Here's how the part is built. I have some questions about the finished solid (model axes, mm). Face numbers are marked on the shaded views. Coordinates: 2 decimals unless noted, no trailing zeros. Loops run counter-clockwise (first coordinate to the right, second up) from the corner with the lowest first, then second, coordinate; pieces in that order, holes last.
```python
from build123d import *

# Parameters (mm, degrees)
F1_DEPTH = 19.5
F3_R     = 3
F4_DEPTH = 60.866634
F3_R_2   = 5
F5_DEPTH = 40.43


with BuildPart() as f1:
    # F0 (on Front) → F1 (new body)
    with BuildSketch(Plane.XZ):
        with BuildLine():
            Line((-53.260562, 35.884366), (-67.116969, 27.884366))
            ThreePointArc((-67.116969, 27.884366), (0, -10.865634), (67.116969, 27.884366))
            Line((67.116969, 27.884366), (53.260562, 35.884366))
            ThreePointArc((53.260562, 35.884366), (0, 5.134366), (-53.260562, 35.884366))
        make_face()
    extrude(amount=F1_DEPTH)

    # F3 (on offset) → F4 (cut, through all)
    with BuildSketch(Plane.XY.offset(50)):
        with Locations((-40, -8.75)):
            Circle(F3_R)
        with Locations((40, -8.75)):
            Circle(F3_R)
    extrude(amount=-F4_DEPTH, mode=Mode.SUBTRACT)

    # F3 (on offset) → F5 (cut)
    with BuildSketch(Plane.XY.offset(50)):
        with Locations((40, -8.75)):
            Circle(F3_R_2)
        with Locations((40, -8.75)):
            Circle(F3_R, mode=Mode.SUBTRACT)
        with Locations((-40, -8.75)):
            Circle(F3_R_2)
        with Locations((-40, -8.75)):
            Circle(F3_R, mode=Mode.SUBTRACT)
    extrude(amount=-F5_DEPTH, mode=Mode.SUBTRACT)


solid = f1.part
```
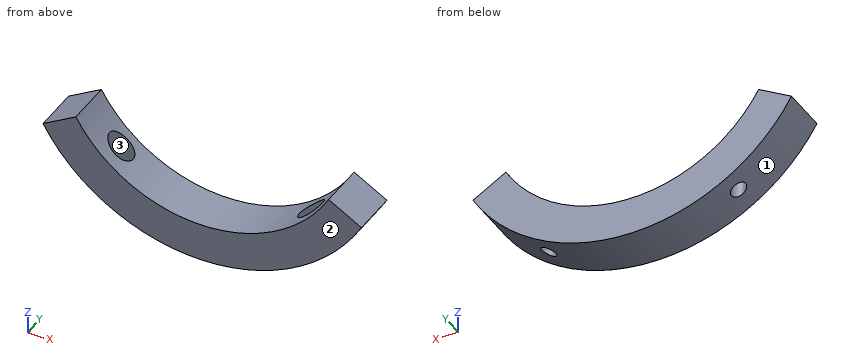
1. I need wall thicknesses on line 1 along Y through (x, z) = (40, 18.25); line 2 along Y through (x, z) = (40, 1); line 3 along X through (y, z) = (-7.5, 19.5). Which ranges of each line are inside material? Lowest first, please.
2. I want a section at B-B (z = 18). Please give me the cut outline in (x, y).
3. I want a section at A-A (x = 41.5). Please give me the cut outline in (y, z).
4. For pin 1 (5 mm diameter, centred on y = -6, z = 20.5, fed in from +X); pin 2 (8 mm diameter, centred on x = 41, y = -10, fed in from +Z); pin 3 (2 mm diameter, centred on y = -6.5, z = 28, fed in from -X); pin 4 (2 mm diameter, centred on x = 29, z = 14, fed in from +Y), each with a flat end and sliding along its axis, tell me the tip position at first contact or that it passes through.
5. We'd pull the mould along X, two halves only. Please class the marked faces 1, 2 and 3: +X half, -X half, draft (parallel to the pull), parting line (faces both ways), or undercut.
6. I want a section at D-D (x = 8). Please give me the cut outline in (y, z).
7. I want a section at C-C (y = -8.75). Please give me the cut outline in (x, z), then the cut area to 3 significant figures.
Response values:
1. line 1: y = -19.5 to -13.75, -3.75 to 0
1. line 2: y = -19.5 to -11.75, -5.75 to 0
1. line 3: x = -61.52 to -44.84, 44.84 to 61.52
2. outline: (-60.34, -19.5) - (-37.64, -19.5) - (-37.64, -13.16) arc R5 cw (long way) to (-37.64, -4.34) - (-37.64, 0) - (-60.34, 0) - close; (37.64, -19.5) - (60.34, -19.5) - (60.34, 0) - (37.64, 0) - (37.64, -4.34) arc R5 cw (long way) to (37.64, -13.16) - close
3. outline: (-19.5, 1.18) - (-11.35, 1.18) - (-11.35, 9.57) - (-13.52, 9.57) - (-13.52, 21.25) - (-19.5, 21.25) - close; (-6.15, 1.18) - (0, 1.18) - (0, 21.25) - (-3.98, 21.25) - (-3.98, 9.57) - (-6.15, 9.57) - close
4. pin 1: stops at x = 64.05
4. pin 2: stops at z = 24.71
4. pin 3: stops at x = -67.12
4. pin 4: passes through
5. face 1: parting line
5. face 2: draft
5. face 3: undercut
6. outline: (-19.5, -10.45) - (0, -10.45) - (0, 5.66) - (-19.5, 5.66) - close
7. outline: (-67.12, 27.88) arc R77.5 ccw to (-43, 2.16) - (-43, 9.57) - (-45, 9.57) - (-45, 24.71) arc R61.5 cw to (-53.26, 35.88) - close; (-37, -1.46) arc R77.5 ccw to (37, -1.46) - (37, 9.57) - (35, 9.57) - (35, 16.07) arc R61.5 cw to (-35, 16.07) - (-35, 9.57) - (-37, 9.57) - close; (43, 2.16) arc R77.5 ccw to (67.12, 27.88) - (53.26, 35.88) arc R61.5 cw to (45, 24.71) - (45, 9.57) - (43, 9.57) - close
7. area: 2,010 mm2
